Check sheet for the modelled part. Datum: model origin and axes. Units: mm. Face numbers are marked on the shaded views. A direction names the side the tool comes from. Round coordinates to 2 decimals unless told otherwise and drop trailing zeros. Write each loop counter-clockwise with the first axis right and the second up, starting at its lowest first coordinate (ties: lowest second). Pieces come first, ordered by that corner, then holes. Notation, with made-up numbers: (5.25, -5) -> (24.25, -5) arc R14 cw to (24.25, 19) -> close; hole circle Ø7 at (37, -13.75). An arc over 180 degrees is marked (long way). Put each result on its own line as item: value. Start each with the question number.
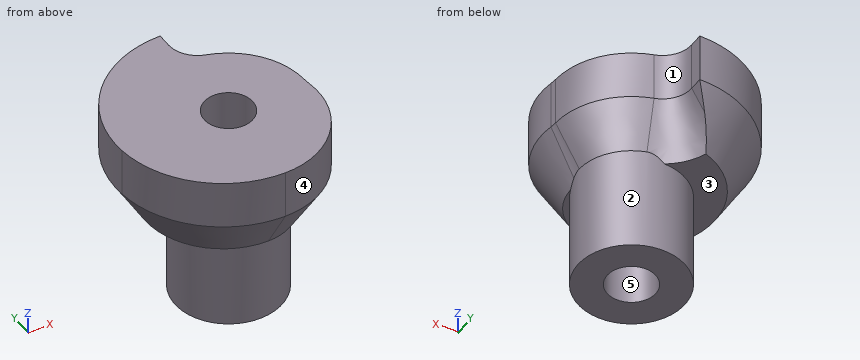
from build123d import *

# Parameters (mm, degrees)
F1_DEPTH      = 10
F2_R          = 5
F3_R          = 3
F4_T1_DEPTH   = 14.3477235542
F4_T4_ANGLE   = 100.2769257202
F4_T6_ANGLE   = 247.4672415992
F4_T8_ANGLE   = 7.8282705893
F4_T10_ANGLE  = 71.7247245492
F4_T12_ANGLE  = 74.1733798681
F5_R          = 5.5
F6_DEPTH      = 10
F6_DEPTH_BACK = 5
F7_R          = 2.5
F8_DEPTH      = 20.0010001


# Not quite as in the source:
# - a fillet or chamfer that OpenCascade refuses, or shapes differently, is made with other operations: its cross-section is extruded or revolved along the edge and cut away or added


with BuildPart() as f1:
    # F0 (on Top) → F1 (new body)
    with BuildSketch(Plane.XY):
        with BuildLine():
            ThreePointArc((0, 11.9994233124), (-8.123630239, 8.4157902443), (-10.9538720645, 0))
            ThreePointArc((-10.9538720645, 0), (-7.4157902443, -7.123630239), (0, -9.9994233124))
            ThreePointArc((0, -9.9994233124), (6.4028990813, -6.9221417854), (8, 0))
            ThreePointArc((8, 0), (5.6568542495, 5.6568542495), (0, 8))
            Line((0, 8), (0, 11.9994233124))
        make_face()
    extrude(amount=F1_DEPTH)

    # F2
    f2_edges = [f1.edges().sort_by_distance(p)[0] for p in [
        (8, 0, 5),
    ]]
    fillet(f2_edges, radius=F2_R)

    # F3
    f3_edges = [f1.edges().sort_by_distance(p)[0] for p in [
        (0, 8, 5),
    ]]
    fillet(f3_edges, radius=F3_R)

    # F4: chamfer of 5 x 3 on 5 edges, made by hand

    # F4_s2 → F4_t1 (cut)
    with BuildSketch(Plane.XZ.offset(-24.9307287984)):
        Polygon((0, 5), (-3, 0), (0, 0), align=None)
    extrude(amount=F4_T1_DEPTH, mode=Mode.SUBTRACT)

    # F4_s3 → F4_t4 (revolve, cut)
    with BuildSketch(Plane.YZ):
        Polygon((-9.9994233124, 5), (-6.9994233124, 0), (-9.9994233124, 0), align=None)
    revolve(axis=Axis((0, -1.7995271056, 0), (0, 0, 1)), revolution_arc=F4_T4_ANGLE, mode=Mode.SUBTRACT)

    # F4_s5 → F4_t6 (revolve, cut)
    with BuildSketch(Plane(origin=(-0.353957442, 0.8531488769, 0), x_dir=(0, 0, 1), z_dir=(0.3832115905, -0.9236605853, 0))):
        Polygon((5, -11.3826349029), (0, -8.3826349029), (0, -11.3826349029), align=None)
    revolve(axis=Axis((0, 1, 0), (0, 0, 1)), revolution_arc=F4_T6_ANGLE, mode=Mode.SUBTRACT)

    # F4_s7 → F4_t8 (revolve, cut)
    with BuildSketch(Plane(origin=(0.315895823, -1.7422505282, 0), x_dir=(0, 0, 1), z_dir=(0.1784059699, -0.9839569655, 0))):
        Polygon((5, -7.8788498285), (0, -4.8788498282), (0, -7.8788498282), align=None)
    revolve(axis=Axis((12.9881297006, 0.5554131457, 0), (0, 0, -1)), revolution_arc=F4_T8_ANGLE, mode=Mode.SUBTRACT)

    # F4_s9 → F4_t10 (revolve, cut)
    with BuildSketch(Plane(origin=(0, 0, 0), x_dir=(0, 0, 1), z_dir=(0.0427240892, -0.9990869092, 0))):
        Polygon((5, -8), (0, -5), (0, -8), align=None)
    revolve(axis=Axis((0, 0, 0), (0, 0, 1)), revolution_arc=F4_T10_ANGLE, mode=Mode.SUBTRACT)

    # F4_s11 → F4_t12 (revolve, cut)
    with BuildSketch(Plane(origin=(0, 0, 0), x_dir=(0, 0, 1), z_dir=(0.9620913858, -0.2727272727, 0))):
        Polygon((5, -8), (0, -5), (0, -8), align=None)
    revolve(axis=Axis((3, 10.5830052443, 0), (0, 0, -1)), revolution_arc=F4_T12_ANGLE, mode=Mode.SUBTRACT)

    # F5 (on face) → F6 (join, two sides)
    with BuildSketch(Plane.XY) as f6_sk:
        Circle(F5_R)
    extrude(amount=-F6_DEPTH)
    extrude(f6_sk.sketch, amount=F6_DEPTH_BACK)

    # F7 (on face) → F8 (cut, through all)
    with BuildSketch(Plane.XY.offset(10)):
        Circle(F7_R)
    extrude(amount=-F8_DEPTH, mode=Mode.SUBTRACT)


solid = f1.part
1. Access from +Z, -Z, +X, -X, +Y, -Y to the whole of each face (thin tool, end or side, straight path). Record for the marked faces 1 and 2.
2. Draft check along X on the marked faces 3, 4 and 5. Enter one of: released by +X, released by -X, zero draft, split by the parting line, or undercut.
3. Gauge pin test, flat ends, axial feed: P1, Ø2, axis at x = -3, z = 5.5, coming from the -Y side; P2, Ø10, axis at y = -0.5, z = -3, coming from the -X side; P3, Ø6, axis at y = -2.5, z = -6.5, coming from the -X side. Record the tip position at first contact, or that the pin passes through.
4. Section check B-B, the plane z = -7.5. Enter the section's corners in (x, y).
5. Section check A-A, the plane z = 3.5. Enter the section's corners in (x, y).
6. Material ranges on L1, parallel to Y at x = 0, z = -0.25; L2, parallel to X at y = 2, z = -2.5; L3, parallel to X at y = 5.5, z = 7.25, recorded low to high. Write a range as [from, to].
Reply:
1. face 1: +Z, -Z, +X, +Y
1. face 2: -Z
2. face 3: zero draft
2. face 4: released by +X
2. face 5: undercut
3. P1: stops at y = -9.82
3. P2: stops at x = -9.13
3. P3: stops at x = -5.5
4. outline: circle Ø11 at (0, 0); hole circle Ø5 at (0, 0)
5. outline: (-0.9, 10.58) -> (-0.9, 11.06) arc R10.1 ccw to (0, -9.1) arc R7.3 ccw to (7.18, -0.5) arc R5.9 cw to (7.09, 0.3) arc R7.1 ccw to (1.94, 6.83) arc R3.9 cw to start; hole circle Ø5 at (0, 0)
6. L1: y = [-5.5, -2.5], [2.5, 5.5]
6. L2: x = [-5.12, -1.5], [1.5, 5.12]
6. L3: x = [-10.04, 5.81]
